The listing builds one solid part. Answer for the finished solid, in the listing's coordinates (mm). A direction names the side the tool comes from. Coordinates: 2 decimals unless noted, no trailing zeros. Order: outer loops, then holes, each group sorted by start corner. A loop starts at its lowest first (then second) coordinate and runs counter-clockwise, first axis right, second up.
```python
from build123d import *

# Parameters (mm, degrees)
CARRIAGE_START                    = 29.8
CARRIAGE_BLOCK_PROFILE_W          = 26
CARRIAGE_BLOCK_PROFILE_H          = 16
CARRIAGE_BLOCK_DEPTH              = 10.6
RAIL_START                        = 29.7
RAIL_RUNNING_CLEARANCE_PROFILE_W  = 26.2
RAIL_RUNNING_CLEARANCE_PROFILE_H  = 9.5
RAIL_RUNNING_CLEARANCE_DEPTH      = 5.55
LONGITUDINAL_START                = 30.65
LONGITUDINAL_GUIDE_KEYS_PROFILE_W = 26
LONGITUDINAL_GUIDE_KEYS_PROFILE_H = 1
LONGITUDINAL_GUIDE_KEYS_DEPTH     = 1.7
CARRIAGE_START_2                  = 36.9
CARRIAGE_SCREW_PILOTS_PROFILE_R   = 0.85
CARRIAGE_SCREW_PILOTS_DEPTH       = 3.6


with BuildPart() as part:
    # Carriage block profile → Carriage block (new body)
    with BuildSketch(Plane.XY.offset(CARRIAGE_START)):
        with Locations((8, 18.5)):
            Rectangle(CARRIAGE_BLOCK_PROFILE_W, CARRIAGE_BLOCK_PROFILE_H)
    extrude(amount=CARRIAGE_BLOCK_DEPTH)

    # Rail running clearance profile → Rail running clearance (cut)
    with BuildSketch(Plane.XY.offset(RAIL_START)):
        with Locations((8, 18.5)):
            Rectangle(RAIL_RUNNING_CLEARANCE_PROFILE_W, RAIL_RUNNING_CLEARANCE_PROFILE_H)
    extrude(amount=RAIL_RUNNING_CLEARANCE_DEPTH, mode=Mode.SUBTRACT)

    # Longitudinal guide keys profile → Longitudinal guide keys (add)
    with BuildSketch(Plane.XY.offset(LONGITUDINAL_START)):
        with Locations((8, 14.15)):
            Rectangle(LONGITUDINAL_GUIDE_KEYS_PROFILE_W, LONGITUDINAL_GUIDE_KEYS_PROFILE_H)
        with Locations((8, 22.85)):
            Rectangle(LONGITUDINAL_GUIDE_KEYS_PROFILE_W, LONGITUDINAL_GUIDE_KEYS_PROFILE_H)
    extrude(amount=LONGITUDINAL_GUIDE_KEYS_DEPTH)

    # Carriage screw pilots profile → Carriage screw pilots (cut)
    with BuildSketch(Plane.XY.offset(CARRIAGE_START_2)):
        with Locations((5, 19.8)):
            Circle(CARRIAGE_SCREW_PILOTS_PROFILE_R)
        with Locations((15, 19.8)):
            Circle(CARRIAGE_SCREW_PILOTS_PROFILE_R)
    extrude(amount=CARRIAGE_SCREW_PILOTS_DEPTH, mode=Mode.SUBTRACT)


solid = part.part
```
(1) Find section C-C (y = 19.8). Write down the section's boundary in (x, z).
(2) Find section B-B (x = 15). Write down the section's boundary in (y, z), and give its area (3 significant figures).
(3) Each of these flat-tipped pins is pushed along its axis until it touches: pin 1 Ø2 at (x, y) = (15, 19.8) entering from -Z; pin 2 Ø7.5 at (x, y) = (5, 17) entering from -Z. Where does it stop, or does it pass through?
(4) For faces 1 (the face through (21, 18, 36)), 2 (the face through (8, 14.65, 31)), 3 (the face through (8, 23, 32.35)), 4 (the face through (15, 20, 36.9)), determine the directions among +Z, -Z, +X, -X, +Y, -Y from which every point of the face is accessible in a straight line to the end or side of a thin tool.
(5) Consider line 1 (X direction, y = 19.8, z = 39.15); line 2 (Y direction, x = 15, z = 38.5); line 3 (Z direction, x = 19.5, y = 14.25). Determine where each line is inside the solid, lowest interval first.
(6) Find section D-D (x = 18.5). Write down the section's boundary in (y, z), and give its area (3 significant figures).
(7) Find section A-A (z = 33). Write down the section's boundary in (x, y).
(8) The mould has two halves that part along Y. Classify faces 5 (the face through (8, 25, 29.8)), 6 (the face through (8, 14, 30.65)), 7 (the face through (8, 26.5, 35)): released by +Y, released by -Y, zero draft, split by the parting line, or undercut.
Findings below:
1. outline: (-5, 35.25) - (21, 35.25) - (21, 40.4) - (15.85, 40.4) - (15.85, 36.9) - (14.15, 36.9) - (14.15, 40.4) - (5.85, 40.4) - (5.85, 36.9) - (4.15, 36.9) - (4.15, 40.4) - (-5, 40.4) - close
2. outline: (10.5, 29.8) - (13.75, 29.8) - (13.75, 30.65) - (14.65, 30.65) - (14.65, 32.35) - (13.75, 32.35) - (13.75, 35.25) - (23.25, 35.25) - (23.25, 32.35) - (22.35, 32.35) - (22.35, 30.65) - (23.25, 30.65) - (23.25, 29.8) - (26.5, 29.8) - (26.5, 40.4) - (20.65, 40.4) - (20.65, 36.9) - (18.95, 36.9) - (18.95, 40.4) - (10.5, 40.4) - close
2. area: 115 mm2
3. pin 1: stops at z = 35.25
3. pin 2: stops at z = 29.8
4. face 1: +Z, -Z, +X, +Y, -Y
4. face 2: -Z, +X, -X
4. face 3: +X, -X
4. face 4: +Z
5. line 1: x = -5 to 4.15, 5.85 to 14.15, 15.85 to 21
5. line 2: y = 10.5 to 18.95, 20.65 to 26.5
5. line 3: z = 30.65 to 32.35, 35.25 to 40.4
6. outline: (10.5, 29.8) - (13.75, 29.8) - (13.75, 30.65) - (14.65, 30.65) - (14.65, 32.35) - (13.75, 32.35) - (13.75, 35.25) - (23.25, 35.25) - (23.25, 32.35) - (22.35, 32.35) - (22.35, 30.65) - (23.25, 30.65) - (23.25, 29.8) - (26.5, 29.8) - (26.5, 40.4) - (10.5, 40.4) - close
6. area: 121 mm2
7. outline: (-5, 10.5) - (21, 10.5) - (21, 13.75) - (-5, 13.75) - close; (-5, 23.25) - (21, 23.25) - (21, 26.5) - (-5, 26.5) - close
8. face 5: zero draft
8. face 6: undercut
8. face 7: released by +Y
